```python
from build123d import *

# Parameters (mm, degrees)
SKETCH1_R           = 0.85
BOSS_EXTRUDE1_DEPTH = 1


with BuildPart() as part:
    # Sketch1 → Boss-Extrude1 (new body)
    with BuildSketch(Plane.XY):
        with BuildLine():
            Line((-2.257442204, -5.86965719), (-2.65, -8.496322734))
            ThreePointArc((-2.65, -8.496322734), (0, 8.9), (2.65, -8.496322734))
            Line((2.65, -8.496322734), (2.257442204, -5.86965719))
            ThreePointArc((2.257442204, -5.86965719), (3.404490458, -3.908136939), (5.56612419, -4.608580375))
            ThreePointArc((5.56612419, -4.608580375), (5.988976647, -4.834574135), (6.407596147, -4.600832621))
            ThreePointArc((6.407596147, -4.600832621), (0, 7), (-6.407596147, -4.600832621))
            ThreePointArc((-6.407596147, -4.600832621), (-5.988976647, -4.834574135), (-5.56612419, -4.608580375))
            ThreePointArc((-5.56612419, -4.608580375), (-3.404490458, -3.908136939), (-2.257442204, -5.86965719))
        make_face()
        with Locations((-4.05, -5.601757633)):
            Circle(SKETCH1_R, mode=Mode.SUBTRACT)
        with Locations((4.05, -5.601757633)):
            Circle(SKETCH1_R, mode=Mode.SUBTRACT)
    extrude(amount=BOSS_EXTRUDE1_DEPTH)


solid = part.part
```
The listing builds one solid part. Answer for the finished solid, in the listing's coordinates (mm). A direction names the side the tool comes from. Round coordinates to 2 decimals unless told otherwise and drop trailing zeros. Loops run counter-clockwise (first coordinate to the right, second up) from the corner with the lowest first, then second, coordinate; pieces in that order, holes last.
1) Consider line 1 (Y direction, x = 4, z = 0.15); line 2 (X direction, y = 4.25, z = 0.6); line 3 (X direction, y = 2.5, z = 0.9). Determine where each line is inside the solid, lowest interval first.
Outcome:
line 1: y = -7.95 to -6.45, -4.75 to -3.79, 5.86 to 7.95
line 2: x = -7.82 to -5.84, 5.84 to 7.82
line 3: x = -8.54 to -6.92, 6.92 to 8.54
2) A cutting plane is placed at D-D on x = 4.05. Determine the outline of the cut face in (y, z).
Outcome:
outline: (-7.93, 0) - (-6.45, 0) - (-6.45, 1) - (-7.93, 1) - close; (-4.75, 0) - (-3.79, 0) - (-3.79, 1) - (-4.75, 1) - close; (5.83, 0) - (7.93, 0) - (7.93, 1) - (5.83, 1) - close
3) Given P1, Ø4, axis at x = 2, y = -2, coming from the +Z side, flat-ended and moving along its own axis, determine where the tip first touches the part or whether it passes through.
Outcome:
P1: passes through
4) A cutting plane is placed at C-C on x = -7.25. Determine the outline of the cut face in (y, z).
Outcome:
outline: (-5.16, 0) - (-2.75, 0) - (-2.75, 1) - (-5.16, 1) - close; (1.61, 0) - (5.16, 0) - (5.16, 1) - (1.61, 1) - close
5) A cutting plane is placed at A-A on y = 4.5. Determine the outline of the cut face in (x, z), plus the area to 3 significant figures.
Outcome:
outline: (-7.68, 0) - (-5.62, 0) - (-5.62, 1) - (-7.68, 1) - close; (5.62, 0) - (7.68, 0) - (7.68, 1) - (5.62, 1) - close
area: 4.11 mm2
6) For faces 1 (the face through (3.3, -4.3, 1)), 2 (the face through (-2.45, -7.16, 0.49)), 3 (the face through (3.37, -3.92, 0.49)), determine the directions among +Z, -Z, +X, -X, +Y, -Y from which every point of the face is accessible in a straight line to the end or side of a thin tool.
Outcome:
face 1: +Z, +X, -X, +Y, -Y
face 2: +Z, -Z, -Y
face 3: +Z, -Z
7) For a pull along Y with two mould halves and no side action, classify faces 4 (the face through (-4.68, -5.03, 0.49)), 5 (the face through (-0.354, 8.893, 0.493)), 6 (the face through (3.3, -4.3, 0)) as released by +Y, released by -Y, zero draft, split by the parting line, or undercut.
Outcome:
face 4: undercut
face 5: split by the parting line
face 6: zero draft
8) A cutting plane is placed at B-B on z = 0.2. Determine the outline of the cut face in (x, y).
Outcome:
outline: (-6.41, -4.6) arc R7.57 cw (long way) to (6.41, -4.6) arc R0.5 cw to (5.57, -4.61) arc R1.81 ccw to (2.26, -5.87) - (2.65, -8.5) arc R8.9 ccw (long way) to (-2.65, -8.5) - (-2.26, -5.87) arc R1.81 ccw to (-5.57, -4.61) arc R0.5 cw to start; hole circle Ø1.7 at (-4.05, -5.6); hole circle Ø1.7 at (4.05, -5.6)
